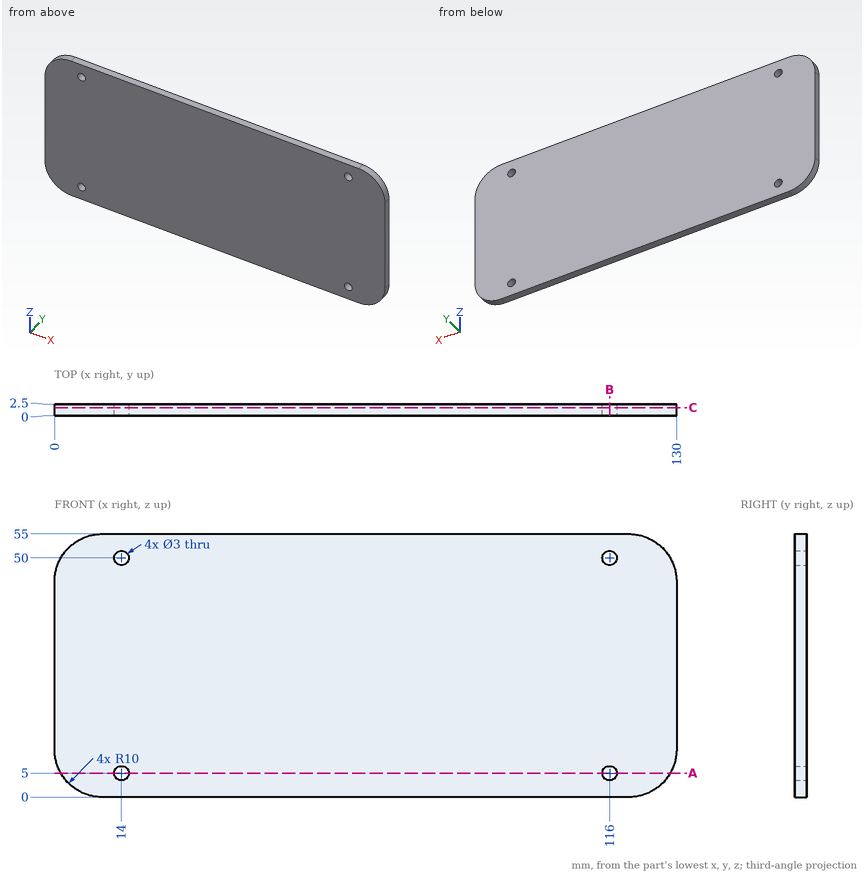
Check sheet for the drawn part. Datum: minimum x, y, z corner. Units: mm. Give positions to 0.01 mm unless a question says otherwise; leave off trailing zeros. Order: outer loops, then holes, each group sorted by start corner. A loop starts at its lowest first (then second) coordinate and runs counter-clockwise, first axis right, second up.
1. Sectioned sample at B-B (x = 116). Record the boundary of the cut face in (y, z), then the cut area to 4 significant figures.
Completed:
outline: (0, 0) - (2.5, 0) - (2.5, 3.5) - (0, 3.5) - close; (0, 6.5) - (2.5, 6.5) - (2.5, 48.5) - (0, 48.5) - close; (0, 51.5) - (2.5, 51.5) - (2.5, 55) - (0, 55) - close
area: 122.5 mm2
2. Sectioned sample at C-C (y = 1.75). Record the boundary of the cut face in (x, z), then the cut area to 3 significant figures.
Completed:
outline: (0, 10) arc R10 ccw to (10, 0) - (120, 0) arc R10 ccw to (130, 10) - (130, 45) arc R10 ccw to (120, 55) - (10, 55) arc R10 ccw to (0, 45) - close; hole circle Ø3 at (14, 5); hole circle Ø3 at (14, 50); hole circle Ø3 at (116, 5); hole circle Ø3 at (116, 50)
area: 7,040 mm2
3. Sectioned sample at A-A (z = 5). Record the boundary of the cut face in (x, y).
Completed:
outline: (1.34, 0) - (12.5, 0) - (12.5, 2.5) - (1.34, 2.5) - close; (15.5, 0) - (114.5, 0) - (114.5, 2.5) - (15.5, 2.5) - close; (117.5, 0) - (128.66, 0) - (128.66, 2.5) - (117.5, 2.5) - close
4. Scan lines: line 1 (Z direction, x = 14, y = 1.35); line 2 (X direction, y = 0.8, z = 5); line 3 (X direction, y = 1, z = 50.5). Record each from-to range of solid material in increasing order.
Completed:
line 1: z = 0 to 3.5, 6.5 to 48.5, 51.5 to 55
line 2: x = 1.34 to 12.5, 15.5 to 114.5, 117.5 to 128.66
line 3: x = 1.65 to 12.59, 15.41 to 114.59, 117.41 to 128.35
